```python
from build123d import *

# Parameters (mm, degrees)
SKETCH1_W           = 139.7
SKETCH1_H           = 114.3
SKETCH1_R           = 9.525
SKETCH1_R_2         = 14.2875
BOSS_EXTRUDE1_DEPTH = 1.5875


with BuildPart() as part:
    # Sketch1 → Boss-Extrude1 (new, symmetric)
    with BuildSketch(Plane(origin=(0, 0, 0), x_dir=(1, 0, 0), z_dir=(0, 1, 0))):
        Rectangle(SKETCH1_W, SKETCH1_H)
        with Locations(Location((0, 43.8912, 0), (0, 0, 270))):
            Circle(SKETCH1_R, mode=Mode.SUBTRACT)
        with Locations(Location((-53.4162, -9.525, 0), (0, 0, 270))):
            Circle(SKETCH1_R, mode=Mode.SUBTRACT)
        with Locations(Location((53.4162, -9.525, 0), (0, 0, 270))):
            Circle(SKETCH1_R, mode=Mode.SUBTRACT)
        with Locations(Location((0, -9.525, 0), (0, 0, 270))):
            Circle(SKETCH1_R_2, mode=Mode.SUBTRACT)
    extrude(amount=BOSS_EXTRUDE1_DEPTH, both=True)


solid = part.part
```
The model under review builds one solid part; all positions refer to its coordinate system, in mm. Coordinates: 2 decimals unless noted, no trailing zeros. Write each loop counter-clockwise with the first axis right and the second up, starting at its lowest first coordinate (ties: lowest second). Pieces come first, ordered by that corner, then holes. Notation, with made-up numbers: (73.5, -24) - (86.5, -24) arc R17 cw to (86.5, -2) - close; hole circle Ø7 at (13.25, 6). An arc over 180 degrees is marked (long way). Answer in a Markdown table with one row per item. Add a question column.
Q1. Consider section C-C on x = -56.5. Give the boundary of the cut face in (y, z), then the cut area to 3 significant figures.
Q2. Draft analysis for pull direction X (two halves, no side actions). For faces 1 (the face through (69.85, 0, 1)), 2 (the face through (-1, 1.588, -14)), 3 (the face through (4.292, -0.022, 23.153)), state which applies: +X half, -X half, draft (parallel to the pull), parting line (faces both ways), or undercut.
Q3. Clearance check with a flat-ended pin moving along its axis: pin 1 (11.5 mm diameter, centred on x = 53.42, z = 9.52, fed in from -Y). State where the tip first meets the part, or that it passes through.
Q4. Consider section B-B on y = 0.45. Give the number of separate pieces and of enclosed holes in the cut face, then the cut area to 3 significant figures.
Q5. Consider section A-A on x = 0. Give the boundary of the cut face in (y, z), then the cut area to 3 significant figures.
Q6. To check wall thickness, follow line 1 along X through (y, z) = (1.1, 5.5); line 2 along X through (y, z) = (0.05, 2.5); line 3 along Z through (x, y) = (3.5, 0.95). State the ranges of each line that lie inside material, in increasing order. Write a range as from..to.
Answers below:
| question | item | result |
|---|---|---|
| 1 | outline | (-1.59, -57.15) - (1.59, -57.15) - (1.59, 0.51) - (-1.59, 0.51) - close; (-1.59, 18.54) - (1.59, 18.54) - (1.59, 57.15) - (-1.59, 57.15) - close |
| 1 | area | 306 mm² |
| 2 | face 1 | +X half |
| 2 | face 2 | draft |
| 2 | face 3 | undercut |
| 3 | pin 1 | through |
| 4 | separate pieces | 1 |
| 4 | enclosed holes | 4 |
| 4 | area | 14,500 mm² |
| 5 | outline | (-1.59, -57.15) - (1.59, -57.15) - (1.59, -53.42) - (-1.59, -53.42) - close; (-1.59, -34.37) - (1.59, -34.37) - (1.59, -4.76) - (-1.59, -4.76) - close; (-1.59, 23.81) - (1.59, 23.81) - (1.59, 57.15) - (-1.59, 57.15) - close |
| 5 | area | 212 mm² |
| 6 | line 1 | -69.85..-62.05, -44.78..-13.71, 13.71..44.78, 62.05..69.85 |
| 6 | line 2 | -69.85..-59.85, -46.98..-12.44, 12.44..46.98, 59.85..69.85 |
| 6 | line 3 | -57.15..-52.75, -35.03..-4.33, 23.38..57.15 |
